Read the model definition and answer for the solid it produces. Units are mm, in the model's axes. A direction names the side the tool comes from. Round coordinates to 2 decimals unless told otherwise and drop trailing zeros. Loops run counter-clockwise (first coordinate to the right, second up) from the corner with the lowest first, then second, coordinate; pieces in that order, holes last. Notation, with made-up numbers: (15, 37.5) -> (58, 37.5) arc R10 ccw to (58, 46.5) -> close; hole circle Ø8 at (-7.5, 24.25). An arc over 180 degrees is marked (long way). Put each result on its own line as item: value.
from build123d import *

# Parameters (mm, degrees)
SKETCH1_R           = 2.5
BOSS_EXTRUDE1_DEPTH = 3
BOSS_EXTRUDE2_DEPTH = 2
FILLET4_R           = 10
SKETCH5_R           = 2
CUT_EXTRUDE1_DEPTH  = 6


with BuildPart() as part:
    # Sketch1 → Boss-Extrude1 (new body)
    with BuildSketch(Plane(origin=(18.3, 0, 0), x_dir=(0, 0, -1), z_dir=(1, 0, 0))):
        with BuildLine():
            Line((61.5, -7.353946086), (61.5, -16.353946086))
            Line((61.5, -16.353946086), (55, -25.353946086))
            Line((55, -25.353946086), (55, -175.353946086))
            Line((55, -175.353946086), (79, -175.353946086))
            Line((79, -175.353946086), (79, -25.353946086))
            Line((79, -25.353946086), (72.5, -16.353946086))
            Line((72.5, -16.353946086), (72.5, -7.353946086))
            ThreePointArc((72.5, -7.353946086), (67, -1.853946086), (61.5, -7.353946086))
        make_face()
        with Locations((67, -7.353946086)):
            Circle(SKETCH1_R, mode=Mode.SUBTRACT)
    extrude(amount=BOSS_EXTRUDE1_DEPTH)

    # Sketch4 → Boss-Extrude2 (add)
    with BuildSketch(Plane.ZY.offset(-18.3)):
        with BuildLine():
            Line((-72, -25.353946086), (-75, -175.353946086))
            Line((-75, -175.353946086), (-59, -175.353946086))
            Line((-59, -175.353946086), (-62, -25.353946086))
            ThreePointArc((-62, -25.353946086), (-67, -20.353946086), (-72, -25.353946086))
        make_face()
    extrude(amount=BOSS_EXTRUDE2_DEPTH)

    # Fillet4
    fillet4_edges = [part.edges().sort_by_distance(p)[0] for p in [
        (19.8, -175.353946086, -55),
        (19.8, -175.353946086, -79),
        (19.8, -25.353946086, -55),
        (19.8, -16.353946086, -61.5),
        (19.8, -25.353946086, -79),
        (19.8, -16.353946086, -72.5),
    ]]
    fillet(fillet4_edges, radius=FILLET4_R)

    # Sketch5 → Cut-Extrude1 (cut, through all)
    with BuildSketch(Plane.ZY.offset(-16.3)):
        with Locations((-67, -127.353946086)):
            Circle(SKETCH5_R)
        with Locations((-67, -167.353946086)):
            Circle(SKETCH5_R)
    extrude(amount=-CUT_EXTRUDE1_DEPTH, mode=Mode.SUBTRACT)


solid = part.part
Item 1: The part is cut by section C-C (y = -121.5). Determine the outline of the cut face in (x, z), then the cut area to 3 significant figures.
Derived:
outline: (16.3, -73.92) -> (18.3, -73.92) -> (18.3, -79) -> (21.3, -79) -> (21.3, -55) -> (18.3, -55) -> (18.3, -60.08) -> (16.3, -60.08) -> close
area: 99.7 mm^2
Item 2: Which of the six approach directions +Z, -Z, +X, -X, +Y, -Y give full straight-line access (tool end or side, diameter ignored) to faces 5 (the cylindrical face through (19.821, -16.155, -72.972)), 6 (the flat face through (20, -10, -61.5)), 7 (the flat face through (18.3, -86, -75))?
Derived:
face 5: -Z, +X, -X, +Y
face 6: +Z, +X, -X, +Y
face 7: -X, +Y
Item 3: Find the intervals of material crossed by line 1 along Y through (x, z) = (19.4, -67); line 2 along Y through (x, z) = (17.95, -67); line 3 along Y through (x, z) = (16.65, -65.75), in increasing order.
Derived:
line 1: y = -175.35 to -169.35, -165.35 to -129.35, -125.35 to -9.85, -4.85 to -1.85
line 2: y = -175.35 to -169.35, -165.35 to -129.35, -125.35 to -20.35
line 3: y = -175.35 to -168.92, -165.79 to -128.92, -125.79 to -20.51
Item 4: Flat-ended cylindrical pins translate along their axes: pin 1 Ø2 at (y, z) = (-69, -74) entering from -X; pin 2 Ø1.5 at (x, z) = (20, -70.5) entering from +Y; pin 3 Ø3 at (y, z) = (-7.35, -67) entering from +X; pin 4 Ø1.5 at (x, y) = (17, -115.5) entering from -Z. Find the tip coordinate at first contact, or state that the pin passes through.
Derived:
pin 1: stops at x = 18.3
pin 2: stops at y = -2.59
pin 3: passes through
pin 4: stops at z = -73.82
Item 5: The part is cut by section B-B (x = 20.3). Determine the outline of the cut face in (y, z).
Derived:
outline: (-175.35, -69) arc R10 ccw to (-165.35, -79) -> (-28.59, -79) arc R10 ccw to (-22.73, -77.11) -> (-18.98, -74.39) arc R10 cw to (-13.12, -72.5) -> (-7.35, -72.5) arc R5.5 ccw to (-7.35, -61.5) -> (-13.12, -61.5) arc R10 cw to (-18.98, -59.61) -> (-22.73, -56.89) arc R10 ccw to (-28.59, -55) -> (-165.35, -55) arc R10 ccw to (-175.35, -65) -> close; hole circle Ø4 at (-167.35, -67); hole circle Ø4 at (-127.35, -67); hole circle Ø5 at (-7.35, -67)
Item 6: The part is cut by section A-A (z = -67). Determine the outline of the cut face in (x, y), then the cut area to 4 significant figures.
Derived:
outline: (16.3, -175.35) -> (21.3, -175.35) -> (21.3, -169.35) -> (16.3, -169.35) -> close; (16.3, -165.35) -> (21.3, -165.35) -> (21.3, -129.35) -> (16.3, -129.35) -> close; (16.3, -125.35) -> (21.3, -125.35) -> (21.3, -9.85) -> (18.3, -9.85) -> (18.3, -20.35) -> (16.3, -20.35) -> close; (18.3, -4.85) -> (21.3, -4.85) -> (21.3, -1.85) -> (18.3, -1.85) -> close
area: 775.5 mm^2
Item 7: For a pull along Y with two mould halves and no side action, classify faces 1 (the cylindrical face through (18.76, -169.13, -66.08)), 2 (the cylindrical face through (19.4, -173.5, -74.8)), 3 (the flat face through (19.779, -20.828, -58.269)), 4 (the flat face through (20, -10, -72.5)) as pulls with the +Y half, pulls with the -Y half, needs draft (parallel to the pull), parting line crosses it, or undercut.
Derived:
face 1: undercut
face 2: pulls with the -Y half
face 3: pulls with the +Y half
face 4: needs draft
Item 8: The part is cut by section D-D (y = -144). Determine the outline of the cut face in (x, z), then the cut area to 3 significant figures.
Derived:
outline: (16.3, -74.37) -> (18.3, -74.37) -> (18.3, -79) -> (21.3, -79) -> (21.3, -55) -> (18.3, -55) -> (18.3, -59.63) -> (16.3, -59.63) -> close
area: 101 mm^2
